```python
from build123d import *
from build123d.topology import SkipClean

# Parameters (mm, degrees)
SKETCH_1_R          = 4.2
EXTRUDE_1_DEPTH     = 10
SKETCH_2_R          = 28.8
EXTRUDE_2_DEPTH     = 10
SKETCH_3_R          = 8.9
EXTRUDE_3_DEPTH     = 20
SKETCH_4_R          = 4.2
CUT_EXTRUDE_1_DEPTH = 59.227484919
CUT_EXTRUDE_2_DEPTH = 47.802136703
SKETCH_8_W          = 6
SKETCH_8_H          = 20.041446809
EXTRUDE_4_DEPTH     = 20
EXTRUDE_5_DEPTH     = 10


with BuildPart() as part:
    # 草图1 → 凸台-拉伸1 (new body)
    with BuildSketch(Plane.XY):
        with BuildLine():
            Line((0, 31), (0, 28.8))
            ThreePointArc((0, 28.8), (28.362463287, 5.001067517), (9.850180128, -27.063147479))
            Line((9.850180128, -27.063147479), (10.602624443, -29.130471244))
            ThreePointArc((10.602624443, -29.130471244), (5.383093508, -30.529040343), (0, -31))
            Line((0, -31), (0, -28.8))
            ThreePointArc((0, -28.8), (-28.362463287, -5.001067517), (-9.850180128, 27.063147479))
            Line((-9.850180128, 27.063147479), (-10.602624443, 29.130471244))
            ThreePointArc((-10.602624443, 29.130471244), (-5.383093508, 30.529040343), (0, 31))
        make_face()
        Circle(SKETCH_1_R, mode=Mode.SUBTRACT)
    extrude(amount=EXTRUDE_1_DEPTH)

    # 草图2 → 凸台-拉伸2 (add)
    with BuildSketch(Plane.XY.offset(10)):
        with Locations(Location((0, 0, 0), (0, 0, 110))):
            Circle(SKETCH_2_R)
    extrude(amount=EXTRUDE_2_DEPTH)

    # 草图3 → 凸台-拉伸3 (add)
    with BuildSketch(Plane.XY.offset(20)):
        Circle(SKETCH_3_R)
    extrude(amount=EXTRUDE_3_DEPTH)

    # 草图4 → 切除-拉伸1 (cut, through all)
    with BuildSketch(Plane.XY.offset(40)):
        Circle(SKETCH_4_R)
    extrude(amount=-CUT_EXTRUDE_1_DEPTH, mode=Mode.SUBTRACT)

    # 草图5 → 切除-拉伸2 (cut, through all)
    with BuildSketch(Plane.XY.offset(20)):
        with BuildLine():
            Line((21.729157013, 14.277385458), (6.847367965, 5.685380546))
            ThreePointArc((6.847367965, 5.685380546), (4.45, 7.707626094), (1.5, 8.77268488))
            Line((1.5, 8.77268488), (1.5, 25.956694705))
            ThreePointArc((1.5, 25.956694705), (13, 22.516660498), (21.729157013, 14.277385458))
        make_face()
        with BuildLine():
            Line((-1.5, 25.956694705), (-1.5, 8.77268488))
            ThreePointArc((-1.5, 8.77268488), (-4.45, 7.707626094), (-6.847367965, 5.685380546))
            Line((-6.847367965, 5.685380546), (-21.729157013, 14.277385458))
            ThreePointArc((-21.729157013, 14.277385458), (-13, 22.516660498), (-1.5, 25.956694705))
        make_face()
        with BuildLine():
            Line((23.229157013, 11.679309247), (8.347367965, 3.087304334))
            ThreePointArc((8.347367965, 3.087304334), (8.9, 0), (8.347367965, -3.087304334))
            Line((8.347367965, -3.087304334), (23.229157013, -11.679309247))
            ThreePointArc((23.229157013, -11.679309247), (26, 0), (23.229157013, 11.679309247))
        make_face()
        with BuildLine():
            Line((21.729157013, -14.277385458), (6.847367965, -5.685380546))
            ThreePointArc((6.847367965, -5.685380546), (4.45, -7.707626094), (1.5, -8.77268488))
            Line((1.5, -8.77268488), (1.5, -25.956694705))
            ThreePointArc((1.5, -25.956694705), (13, -22.516660498), (21.729157013, -14.277385458))
        make_face()
        with BuildLine():
            Line((-1.5, -25.956694705), (-1.5, -8.77268488))
            ThreePointArc((-1.5, -8.77268488), (-4.45, -7.707626094), (-6.847367965, -5.685380546))
            Line((-6.847367965, -5.685380546), (-21.729157013, -14.277385458))
            ThreePointArc((-21.729157013, -14.277385458), (-13, -22.516660498), (-1.5, -25.956694705))
        make_face()
        with BuildLine():
            Line((-23.229157013, -11.679309247), (-8.347367965, -3.087304334))
            ThreePointArc((-8.347367965, -3.087304334), (-8.9, 0), (-8.347367965, 3.087304334))
            Line((-8.347367965, 3.087304334), (-23.229157013, 11.679309247))
            ThreePointArc((-23.229157013, 11.679309247), (-26, 0), (-23.229157013, -11.679309247))
        make_face()
    extrude(amount=-CUT_EXTRUDE_2_DEPTH, mode=Mode.SUBTRACT)

    # 草图8 → 凸台-拉伸4 (add)
    with BuildSketch(Plane.XY.offset(20)):
        with Locations((0, 17.104380285)):
            Rectangle(SKETCH_8_W, SKETCH_8_H)
    extrude(amount=-EXTRUDE_4_DEPTH)

    # 草图9 → 凸台-拉伸5 (add)
    with SkipClean():  # the faces are left unmerged after this step: merging them gives an invalid solid
        with BuildSketch(Plane.XY.offset(20)):
            with BuildLine():
                Line((-3, 28.643323829), (-3, 11.101801656))
                ThreePointArc((-3, 11.101801656), (0, 11.5), (3, 11.101801656))
                Line((3, 11.101801656), (3, 28.643323829))
                ThreePointArc((3, 28.643323829), (0, 28.8), (-3, 28.643323829))
            make_face()
        extrude(amount=EXTRUDE_5_DEPTH)


solid = part.part
```
Verification items for the finished model (mm, model axes). A direction names the side the tool comes from. Coordinates: 2 decimals unless noted, no trailing zeros. Loops run counter-clockwise (first coordinate to the right, second up) from the corner with the lowest first, then second, coordinate; pieces in that order, holes last. Notation, with made-up numbers: (50.5, 47.5) -> (75.5, 47.5) arc R20 ccw to (75.5, 60.5) -> close; hole circle Ø6 at (18, 79). An arc over 180 degrees is marked (long way). Answer in a Markdown table with one row per item.
1) Scan lines: line 1 along Y through (x, z) = (0, 11); line 2 along X through (y, z) = (-1, 12); line 3 along Y through (x, z) = (-18, 9.5). Record each from-to range of solid material in increasing order. Write a range as from..to.
The answers:
| item | result |
|---|---|
| line 1 | y = -28.8..-4.2, 4.2..28.8 |
| line 2 | x = -28.78..-25.98, -8.84..-4.08, 4.08..8.84, 25.98..28.78 |
| line 3 | y = -22.48..-18.76, -12.12..-8.66, 8.66..12.12, 18.76..22.48 |
2) Access from +Z, -Z, +X, -X, +Y, -Y to the whole of each face (thin tool, end or side, straight path). Record for faces 1 (the face through (10.22, -28.08, 4.93)), 2 (the face through (-13.15, -22.43, 10.14)), 3 (the face through (0, 11.5, 24.9)), 4 (the face through (0, 20, 30)).
The answers:
| item | result |
|---|---|
| face 1 | +Z, -Z, +X |
| face 2 | +Z, -Z |
| face 3 | +Z |
| face 4 | +Z, +X, -X, +Y |
3) Section check B-B (z = 25). Record the cut outline in (x, y), and give its area (3 significant figures).
The answers:
| item | result |
|---|---|
| outline | circle Ø17.8 at (0, 0); (-3, 11.1) arc R11.5 cw to (3, 11.1) -> (3, 28.64) arc R28.8 ccw to (-3, 28.64) -> close; hole circle Ø8.4 at (0, 0) |
| area | 298 mm2 |
4) Section check D-D (y = -10). Record the cut outline in (x, z).
The answers:
| item | result |
|---|---|
| outline | (-27.01, 0) -> (-24, 0) -> (-24, 20) -> (-27.01, 20) -> close; (-20.32, 0) -> (-14.32, 0) -> (-14.32, 20) -> (-20.32, 20) -> close; (-1.5, 0) -> (1.5, 0) -> (1.5, 20) -> (-1.5, 20) -> close; (14.32, 0) -> (20.32, 0) -> (20.32, 20) -> (14.32, 20) -> close; (24, 0) -> (27.01, 0) -> (27.01, 20) -> (24, 20) -> close |
5) Section check C-C (x = 15). Record the cut outline in (y, z), and give its area (3 significant figures).
The answers:
| item | result |
|---|---|
| outline | (-24.59, 0) -> (-21.24, 0) -> (-21.24, 20) -> (-24.59, 20) -> close; (-10.39, 0) -> (-6.93, 0) -> (-6.93, 20) -> (-10.39, 20) -> close; (6.93, 0) -> (10.39, 0) -> (10.39, 20) -> (6.93, 20) -> close; (21.24, 0) -> (24.59, 0) -> (24.59, 20) -> (21.24, 20) -> close |
| area | 273 mm2 |
6) Section check A-A (y = 0). Record the cut outline in (x, z).
The answers:
| item | result |
|---|---|
| outline | (-28.8, 0) -> (-26, 0) -> (-26, 20) -> (-28.8, 20) -> close; (-8.9, 0) -> (-4.2, 0) -> (-4.2, 40) -> (-8.9, 40) -> close; (4.2, 0) -> (8.9, 0) -> (8.9, 40) -> (4.2, 40) -> close; (26, 0) -> (28.8, 0) -> (28.8, 20) -> (26, 20) -> close |
7) Depth check by flat-ended pin: P1, Ø12, axis at x = -14.5, y = 13.5, coming from the +Z side; P2, Ø8.5, axis at y = -14.5, z = 5.5, coming from the -X side; P3, Ø10, axis at x = -2.5, z = 24.5, coming from the +Y side; P4, Ø9.5, axis at x = 0, y = 0, coming from the +Z side. Enter the tip coordinate at first touch or a pass-through.
The answers:
| item | result |
|---|---|
| P1 | stops at z = 20 |
| P2 | stops at x = -26.91 |
| P3 | stops at y = 28.8 |
| P4 | stops at z = 40 |
8) Draft check along Y on faces 5 (the face through (14.39, 10.04, 10.14)), 6 (the face through (4.006, 1.262, 19.72)), 7 (the face through (5, -29, 10)). Enter one of: released by +Y, released by -Y, zero draft, split by the parting line, or undercut.
The answers:
| item | result |
|---|---|
| face 5 | undercut |
| face 6 | undercut |
| face 7 | zero draft |
